from build123d import *

# Parameters (mm, degrees)
SKETCH1_R            = 4.826
BOSS_EXTRUDE1_DEPTH  = 22.225
CUT_EXTRUDE2_DEPTH   = 45.45
CUT_EXTRUDE3_DEPTH   = 45.45
FILLET1_R            = 2.54
CUT_EXTRUDE4_DEPTH   = 56.5625
MIRROR3_COPY_1_DEPTH = 56.5625


with BuildPart() as part:
    # Sketch1 → Boss-Extrude1 (new body, symmetric)
    with BuildSketch(Plane.XY):
        Polygon((-25.4, 72.8218), (25.4, 72.8218), (25.4, -72.8218), (-25.4, -72.8218), (-25.4, -76.2), (-30.1625, -76.2), (-30.1625, 76.2), (-25.4, 76.2), align=None)
        with Locations((0, 57.15)):
            Circle(SKETCH1_R, mode=Mode.SUBTRACT)
        with Locations((0, -57.15)):
            Circle(SKETCH1_R, mode=Mode.SUBTRACT)
    extrude(amount=BOSS_EXTRUDE1_DEPTH, both=True)

    # Sketch3 → Cut-Extrude2 (cut, through all)
    with BuildSketch(Plane.XY.offset(22.225)):
        with BuildLine():
            Line((-19.05, 66.4718), (-9.525, 66.4718))
            Line((-9.525, 66.4718), (-9.525, 57.15))
            ThreePointArc((-9.525, 57.15), (0, 47.625), (9.525, 57.15))
            Line((9.525, 57.15), (9.525, 66.4718))
            Line((9.525, 66.4718), (19.05, 66.4718))
            Line((19.05, 66.4718), (19.05, 0))
            Line((19.05, 0), (-19.05, 0))
            Line((-19.05, 0), (-19.05, 66.4718))
        make_face()
    cut_extrude2 = extrude(amount=-CUT_EXTRUDE2_DEPTH, mode=Mode.SUBTRACT)

    # Sketch4 → Cut-Extrude3 (cut, through all)
    with BuildSketch(Plane.XY.offset(22.225)):
        with BuildLine():
            Line((-22.225, 72.8218), (-25.4, 72.8218))
            ThreePointArc((-25.4, 72.8218), (-23.8125, 71.2343), (-22.225, 72.8218))
        make_face()
    cut_extrude3 = extrude(amount=-CUT_EXTRUDE3_DEPTH, mode=Mode.SUBTRACT)

    # Mirror1: Cut-Extrude2, Cut-Extrude3 across plane
    add(cut_extrude2.mirror(Plane.ZX), mode=Mode.SUBTRACT)
    add(cut_extrude3.mirror(Plane.ZX), mode=Mode.SUBTRACT)

    # Fillet1
    fillet1_edges = [part.edges().sort_by_distance(p)[0] for p in [
        (25.4, 72.8218, 0),
        (25.4, -72.8218, 0),
        (-30.1625, -76.2, 0),
        (-30.1625, 76.2, 0),
        (-19.05, 66.4718, 0),
        (-9.525, 66.4718, 0),
        (9.525, 66.4718, 0),
        (19.05, 66.4718, 0),
        (-19.05, -66.4718, 0),
        (19.05, -66.4718, 0),
        (9.525, -66.4718, 0),
        (-9.525, -66.4718, 0),
    ]]
    fillet(fillet1_edges, radius=FILLET1_R)

    # Sketch5 → Cut-Extrude4 (cut, through all)
    with BuildSketch(Plane(origin=(25.4, 0, 0), x_dir=(0, 0, -1), z_dir=(1, 0, 0))):
        Polygon((16.3068, 76.2), (22.225, 70.2818), (22.225, 76.2), align=None)
    cut_extrude4 = extrude(amount=-CUT_EXTRUDE4_DEPTH, mode=Mode.SUBTRACT)

    # Mirror2: Cut-Extrude4 across plane
    add(cut_extrude4.mirror(Plane.XY), mode=Mode.SUBTRACT)

    # Mirror3: Cut-Extrude4 across plane
    add(cut_extrude4.mirror(Plane.ZX), mode=Mode.SUBTRACT)

    # Mirror3 copy 1 sketch → Mirror3 copy 1 (cut, through all)
    with BuildSketch(Plane(origin=(25.4, 0, 0), x_dir=(0, 0, 1), z_dir=(1, 0, 0))):
        Polygon((16.3068, 76.2), (22.225, 70.2818), (22.225, 76.2), align=None)
    extrude(amount=-MIRROR3_COPY_1_DEPTH, mode=Mode.SUBTRACT)


solid = part.part
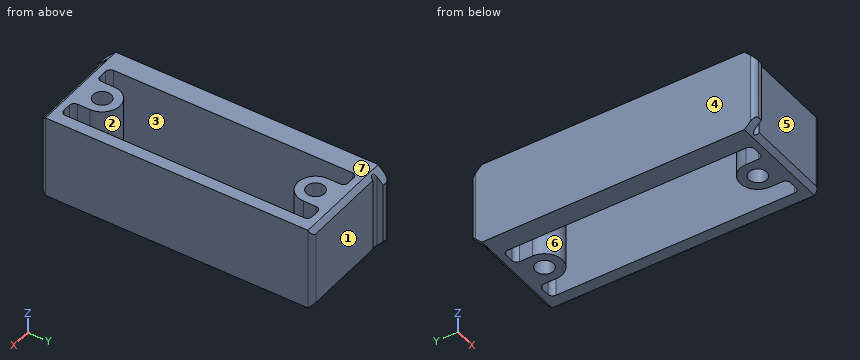
Read the model definition and answer for the solid it produces. Units are mm, in the model's axes. Face numbers are marked on the shaded views. A direction names the side the tool comes from. Coordinates: 2 decimals unless noted, no trailing zeros. Order: outer loops, then holes, each group sorted by start corner. A loop starts at its lowest first (then second) coordinate and runs counter-clockwise, first axis right, second up. Notation, with made-up numbers: (73, 56.5) - (132, 56.5) arc R21 ccw to (132, 93.5) - close; hole circle Ø5 at (17, -35.75). An arc over 180 degrees is marked (long way). Use one line per item in the form item = value.
(1) Section A-A, the plane x = 0 is taken. Give the vertices of the cut face in (y, z) (3 decimals).
Computed values:
outline = (-72.822, -19.685) - (-70.282, -22.225) - (-61.976, -22.225) - (-61.976, 22.225) - (-70.282, 22.225) - (-72.822, 19.685) - close; (-52.324, -22.225) - (-47.625, -22.225) - (-47.625, 22.225) - (-52.324, 22.225) - close; (47.625, -22.225) - (52.324, -22.225) - (52.324, 22.225) - (47.625, 22.225) - close; (61.976, -22.225) - (70.282, -22.225) - (72.822, -19.685) - (72.822, 19.685) - (70.282, 22.225) - (61.976, 22.225) - close
(2) Which of the six approach directions +Z, -Z, +X, -X, +Y, -Y give full straight-line access (tool end or side, diameter ignored) to the marked faces 5, 6 and 7?
Computed values:
face_5 = +Z, -Z, +X, -Y
face_6 = +Z, -Z
face_7 = +Z, +X, -X, +Y, -Y
(3) For a pull along Y with two mould halves and no side action, classify the marked faces 1, 2, 3 and 4 as pulls with the +Y half, pulls with the -Y half, needs draft (parallel to the pull), parting line crosses it, or undercut.
Computed values:
face_1 = pulls with the +Y half
face_2 = undercut
face_3 = undercut
face_4 = needs draft
(4) Section C-C, the plane z = -0.5 is taken. Give the number of separate pieces and of enclosed holes in the cut face, then the cut area to 3 significant figures.
Computed values:
separate_pieces = 1
enclosed_holes = 3
area = 3,550 mm²
(5) Given pin 1 Ø10 at (x, z) = (-14.5, 1) entering from +Y; pin 2 Ø12 at (x, z) = (-9.5, 8.5) entering from -Y; pin 3 Ø3.5 at (y, z) = (-74, -7) entering from +X; pin 4 Ø7.5 at (x, y) = (0, 57.15) entering from -Z, each flat-ended and moving along its own axis, determine where each tip first touches the part or whether it passes through.
Computed values:
pin_1 = 72.82
pin_2 = -72.82
pin_3 = 24.47
pin_4 = through
(6) Straight lines are drawn through the part: L1, parallel to X at y = -57, z = -3; L2, parallel to Y at x = 0, z = -7.5 (3 decimals); L3, parallel to X at y = 29, z = 4. For each, find the intervals that lie inside material, in ascending order.
Computed values:
L1 = -30.16 to -19.05, -9.52 to -4.82, 4.82 to 9.52, 19.05 to 25.4
L2 = -72.822 to -61.976, -52.324 to -47.625, 47.625 to 52.324, 61.976 to 72.822
L3 = -30.16 to -19.05, 19.05 to 25.4
